```python
from build123d import *

# Parameters (mm, degrees)
F1_DEPTH = 30
F2_W     = 3
F2_H     = 25
F2_W_2   = 12
F2_H_2   = 10.5
F2_W_3   = 9.15
F2_H_3   = 11.2
F2_W_4   = 52.23
F2_H_4   = 10
F3_DEPTH = 14.001
F5_D     = 3.3
F6_R     = 3


with BuildPart() as f1:
    # F0 (on Top) → F1 (new body, symmetric)
    with BuildSketch(Plane.XY):
        with BuildLine():
            Line((-52.5, 0), (52.5, 0))
            ThreePointArc((52.5, 0), (53.2071067812, -0.2928932188), (53.5, -1))
            Line((53.5, -1), (53.5, -12))
            Line((53.5, -12), (55.5, -12))
            Line((55.5, -12), (55.5, -1))
            ThreePointArc((55.5, -1), (54.6213203436, 1.1213203436), (52.5, 2))
            Line((52.5, 2), (-52.5, 2))
            ThreePointArc((-52.5, 2), (-54.6213203436, 1.1213203436), (-55.5, -1))
            Line((-55.5, -1), (-55.5, -12))
            Line((-55.5, -12), (-53.5, -12))
            Line((-53.5, -12), (-53.5, -1))
            ThreePointArc((-53.5, -1), (-53.2071067812, -0.2928932188), (-52.5, 0))
        make_face()
    extrude(amount=F1_DEPTH, both=True)

    # F2 (on face) → F3 (cut, through all)
    with BuildSketch(Plane(origin=(0, 2, 0), x_dir=(-1, 0, 0), z_dir=(0, 1, 0))):
        with Locations((-54, 0)):
            Rectangle(F2_W, F2_H)
        with Locations((54, 0)):
            Rectangle(F2_W, F2_H)
        with Locations((-15.81, 19.1)):
            Rectangle(F2_W_2, F2_H_2)
        with Locations((14.385, 18.75)):
            Rectangle(F2_W_3, F2_H_3)
        with Locations((1.505, 6.55)):
            Rectangle(F2_W_4, F2_H_4)
    extrude(amount=-F3_DEPTH, mode=Mode.SUBTRACT)

    # F5 (through all)
    with Locations(Plane.YZ.offset(55.5)):
        with Locations((-6.5, 21.25), (-6.5, -21.25)):
            Hole(F5_D / 2)

    # F6
    f6_edges = [f1.edges().sort_by_distance(p)[0] for p in [
        (-54.5, -12, 30),
        (-54.5, -12, 12.5),
        (-54.5, -12, -12.5),
        (-54.5, -12, -30),
        (54.5, -12, 30),
        (54.5, -12, 12.5),
        (54.5, -12, -12.5),
        (54.5, -12, -30),
    ]]
    fillet(f6_edges, radius=F6_R)


solid = f1.part
```
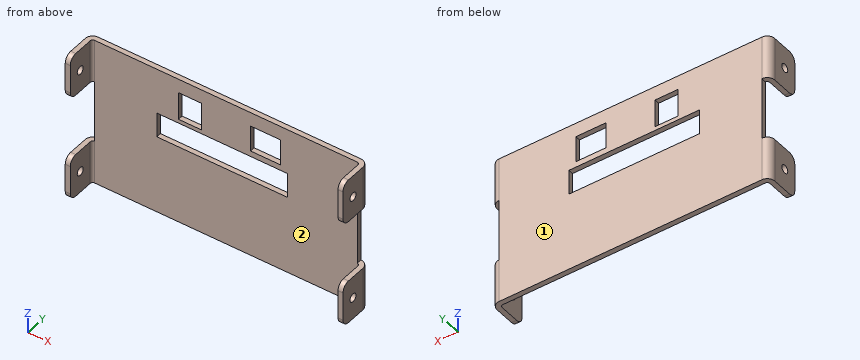
Verification items for the finished model (mm, model axes). Face numbers are marked on the shaded views. Give positions to 0.01 mm unless a question says otherwise; leave off trailing zeros. Order: outer loops, then holes, each group sorted by start corner. A loop starts at its lowest first (then second) coordinate and runs counter-clockwise, first axis right, second up. Notation, with made-up numbers: (60, -9) - (110, -9) arc R7 cw to (110, -1) - close; hole circle Ø10 at (77, 7). An arc over 180 degrees is marked (long way). Answer as CSV lines item,"result". Start each with the question number.
Item 1: Section check B-B, the plane x = 20. Record the boundary of the cut face in (y, z), plus the area to 3 significant figures.
Item 2: Section check D-D, the plane z = -21.25. Record the boundary of the cut face in (x, y), plus the area to 3 significant figures.
Item 3: Section check A-A, the plane z = 21.25. Record the boundary of the cut face in (x, y), plus the area to 3 significant figures.
Item 4: Gauge pin test, flat ends, axial feed: pin 1 (1.6 mm diameter, centred on y = 0.5, z = 20.5, fed in from +X); pin 2 (2 mm diameter, centred on y = 1.5, z = 8.5, fed in from -X); pin 3 (4.5 mm diameter, centred on y = -6.5, z = -21.25, fed in from -X); pin 4 (1.6 mm diameter, centred on y = 1, z = 9, fed in from +X). Record the tip position at first contact, or that the pin passes through.
Item 5: Mould release check, pull along X, two halves, no side actions. Record for the marked faces 1 and 2: released by +X, released by -X, zero draft, split by the parting line, or undercut.
Item 6: Material ranges on L1, parallel to Z at x = 54.05, y = -6.5; L2, parallel to Z at x = 21.5, y = 1; L3, parallel to X at y = -3.5, z = 19.5, recorded low to high.
Item 7: Section check C-C, the plane y = -6.5. State how many separate pieces and enclosed holes the cut face has, plus the area to 3 significant figures.
Filled in:
1,outline,"(0, -30) - (2, -30) - (2, 1.55) - (0, 1.55) - close; (0, 11.55) - (2, 11.55) - (2, 13.85) - (0, 13.85) - close; (0, 24.35) - (2, 24.35) - (2, 30) - (0, 30) - close"
1,area,"79.0 mm^2"
2,outline,"(-55.5, -12) - (-53.5, -12) - (-53.5, -8.15) - (-55.5, -8.15) - close; (-55.5, -4.85) - (-53.5, -4.85) - (-53.5, -1) arc R1 cw to (-52.5, 0) - (52.5, 0) arc R1 cw to (53.5, -1) - (53.5, -4.85) - (55.5, -4.85) - (55.5, -1) arc R3 ccw to (52.5, 2) - (-52.5, 2) arc R3 ccw to (-55.5, -1) - close; (53.5, -12) - (55.5, -12) - (55.5, -8.15) - (53.5, -8.15) - close"
2,area,"253 mm^2"
3,outline,"(-55.5, -12) - (-53.5, -12) - (-53.5, -8.15) - (-55.5, -8.15) - close; (-55.5, -4.85) - (-53.5, -4.85) - (-53.5, -1) arc R1 cw to (-52.5, 0) - (-18.96, 0) - (-18.96, 2) - (-52.5, 2) arc R3 ccw to (-55.5, -1) - close; (-9.81, 0) - (9.81, 0) - (9.81, 2) - (-9.81, 2) - close; (21.81, 0) - (52.5, 0) arc R1 cw to (53.5, -1) - (53.5, -4.85) - (55.5, -4.85) - (55.5, -1) arc R3 ccw to (52.5, 2) - (21.81, 2) - close; (53.5, -12) - (55.5, -12) - (55.5, -8.15) - (53.5, -8.15) - close"
3,area,"211 mm^2"
4,pin 1,"x = 55.42"
4,pin 2,"x = -52.5"
4,pin 3,"x = -55.5"
4,pin 4,"x = 52.5"
5,face 1,"zero draft"
5,face 2,"undercut"
6,L1,"-30 to -22.9, -19.6 to -12.5, 12.5 to 19.6, 22.9 to 30"
6,L2,"-30 to 1.55, 11.55 to 13.85, 24.35 to 30"
6,L3,"-55.5 to -53.5, 53.5 to 55.5"
7,separate pieces,"8"
7,enclosed holes,"0"
7,area,"114 mm^2"
